Source: CAD feature listing. Evaluate the final solid. Frame: model axes, mm. A direction names the side the tool comes from. Give positions to 0.01 mm unless a question says otherwise; leave off trailing zeros. Order: outer loops, then holes, each group sorted by start corner. A loop starts at its lowest first (then second) coordinate and runs counter-clockwise, first axis right, second up.
1) Section C-C, the plane x = -22. Return loops of the section in (y, z).
2) Section B-B, the plane z = -14. Return loops of the section in (x, y).
3) Section D-D, the plane z = 3. Return loops of the section in (x, y).
4) Material intervals for line 1 (Y direction, x = 19.25, z = 0); line 2 (Z direction, x = 22, y = -14.5); line 3 (Y direction, x = 3, z = 0), sorted ascending.
5) Access query for faces 1 (the face through (-24.25, 18.2, 18.2)), 2 (the face through (19.18, 30.686, -0.221)). Directions: +Z, -Z, +X, -X, +Y, -Y. A direction counts if a zero-diameter tool reaches every point of the face in a straight line with its end or side. Return the directions, or none.
6) First-contact query: P1, Ø8, axis at x = -18.5, y = 17, coming from the -Z side; P2, Ø2, axis at x = -2, z = 1, coming from the -Y side; P3, Ø10.5, axis at y = 13, z = 15.5, coming from the -X side; P4, Ø4, axis at y = -29, z = 0, coming from the +X side. Flat tips, straight axial feed; report the tip coordinate or a pass-through.
7) Draft query along Z for faces 3 (the face through (19.18, 12.99, -24.33)), 4 (the face through (13.406, -28.707, 0.038)). Return one class per face: released by +Z, released by -Z, zero draft, split by the parting line, or undercut.
8) Section A-A, the plane y = -7. Return loops of the section in (x, z), plus the area to 3 significant figures.
```python
from build123d import *

# Parameters (mm, degrees)
CROQUIS1_R                       = 32.7
CROQUIS1_R_2                     = 21
SALIENTE_EXTRUIR1_DEPTH          = 24.25
CROQUIS3_R                       = 32.7
SALIENTE_EXTRUIR3_DEPTH          = 5
CROQUIS4_R                       = 3.5
CORTAR_EXTRUIR1_DEPTH            = 6
TALADRO_DE_MARGEN_PARA_M31_D     = 3.4
TALADRO_DE_MARGEN_PARA_M31_DEPTH = 10
TALADRO_DE_MARGEN_PARA_M31_TIP   = 1.021463052


with BuildPart() as part:
    # Croquis1 → Saliente-Extruir1 (new, symmetric)
    with BuildSketch(Plane(origin=(0, 0, 0), x_dir=(0, 0, -1), z_dir=(1, 0, 0))):
        with Locations(Location((0, 0, 0), (0, 0, 180))):
            Circle(CROQUIS1_R)
        with Locations(Location((0, 0, 0), (0, 0, 180))):
            Circle(CROQUIS1_R_2, mode=Mode.SUBTRACT)
    extrude(amount=SALIENTE_EXTRUIR1_DEPTH, both=True)

    # Croquis3 → Saliente-Extruir3 (add)
    with BuildSketch(Plane.ZY.offset(24.25)):
        Circle(CROQUIS3_R)
        with BuildLine():
            Line((-18, -21), (18, -21))
            ThreePointArc((18, -21), (20.121320344, -20.121320344), (21, -18))
            Line((21, -18), (21, 18))
            ThreePointArc((21, 18), (20.121320344, 20.121320344), (18, 21))
            Line((18, 21), (-18, 21))
            ThreePointArc((-18, 21), (-20.121320344, 20.121320344), (-21, 18))
            Line((-21, 18), (-21, -18))
            ThreePointArc((-21, -18), (-20.121320344, -20.121320344), (-18, -21))
        make_face(mode=Mode.SUBTRACT)
    extrude(amount=SALIENTE_EXTRUIR3_DEPTH)

    # Croquis4 → Cortar-Extruir1 (cut)
    with BuildSketch(Plane.ZY.offset(24.25)):
        with Locations((15.5, 15.5)):
            Circle(CROQUIS4_R)
        with Locations((-15.5, 15.5)):
            Circle(CROQUIS4_R)
        with Locations((-15.5, -15.5)):
            Circle(CROQUIS4_R)
        with Locations((15.5, -15.5)):
            Circle(CROQUIS4_R)
    extrude(amount=-CORTAR_EXTRUIR1_DEPTH, mode=Mode.SUBTRACT)

    # Taladro de margen para M31
    with Locations(Plane(origin=(24.25, 0, 0), x_dir=(0, 0, -1), z_dir=(1, 0, 0))):
        with Locations((0, 29), (25.11473671, 14.5), (25.11473671, -14.5), (0, -29), (-25.11473671, -14.5), (-25.11473671, 14.5)):
            Hole(TALADRO_DE_MARGEN_PARA_M31_D / 2, depth=TALADRO_DE_MARGEN_PARA_M31_DEPTH)
            with Locations((0, 0, -(TALADRO_DE_MARGEN_PARA_M31_DEPTH + TALADRO_DE_MARGEN_PARA_M31_TIP / 2))):  # 118° drill point
                Cone(0, TALADRO_DE_MARGEN_PARA_M31_D / 2, TALADRO_DE_MARGEN_PARA_M31_TIP, mode=Mode.SUBTRACT)


solid = part.part
```
From the geometry:
1. outline: circle Ø65.4 at (0, 0); hole (-17, -12.34) arc R3.5 ccw (long way) to (-12.34, -17) arc R21 ccw to (12.34, -17) arc R3.5 ccw (long way) to (17, -12.34) arc R21 ccw to (17, 12.34) arc R3.5 ccw (long way) to (12.34, 17) arc R21 ccw to (-12.34, 17) arc R3.5 ccw (long way) to (-17, 12.34) arc R21 ccw to start
2. outline: (-29.25, -29.55) - (24.25, -29.55) - (24.25, -15.65) - (-18.25, -15.65) - (-18.25, -18.66) - (-24.25, -18.66) - (-24.25, -21) - (-29.25, -21) - close; (-29.25, 21) - (-24.25, 21) - (-24.25, 18.66) - (-18.25, 18.66) - (-18.25, 15.65) - (24.25, 15.65) - (24.25, 29.55) - (-29.25, 29.55) - close
3. outline: (-29.25, -32.56) - (24.25, -32.56) - (24.25, -20.78) - (-24.25, -20.78) - (-24.25, -21) - (-29.25, -21) - close; (-29.25, 21) - (-24.25, 21) - (-24.25, 20.78) - (24.25, 20.78) - (24.25, 32.56) - (-29.25, 32.56) - close
4. line 1: y = -32.7 to -30.7, -27.3 to -21, 21 to 27.3, 30.7 to 32.7
4. line 2: z = -29.31 to -26.81, -23.41 to -15.19, 15.19 to 23.41, 26.81 to 29.31
4. line 3: y = -32.7 to -21, 21 to 32.7
5. face 1: -X
5. face 2: +X
6. P1: stops at z = -30
6. P2: stops at y = -32.7
6. P3: stops at x = -24.25
6. P4: stops at x = 24.25
7. face 3: undercut
7. face 4: undercut
8. outline: (-29.25, -31.94) - (24.25, -31.94) - (24.25, -19.8) - (-24.25, -19.8) - (-24.25, -21) - (-29.25, -21) - close; (-29.25, 21) - (-24.25, 21) - (-24.25, 19.8) - (24.25, 19.8) - (24.25, 31.94) - (-29.25, 31.94) - close
8. area: 1,290 mm2
